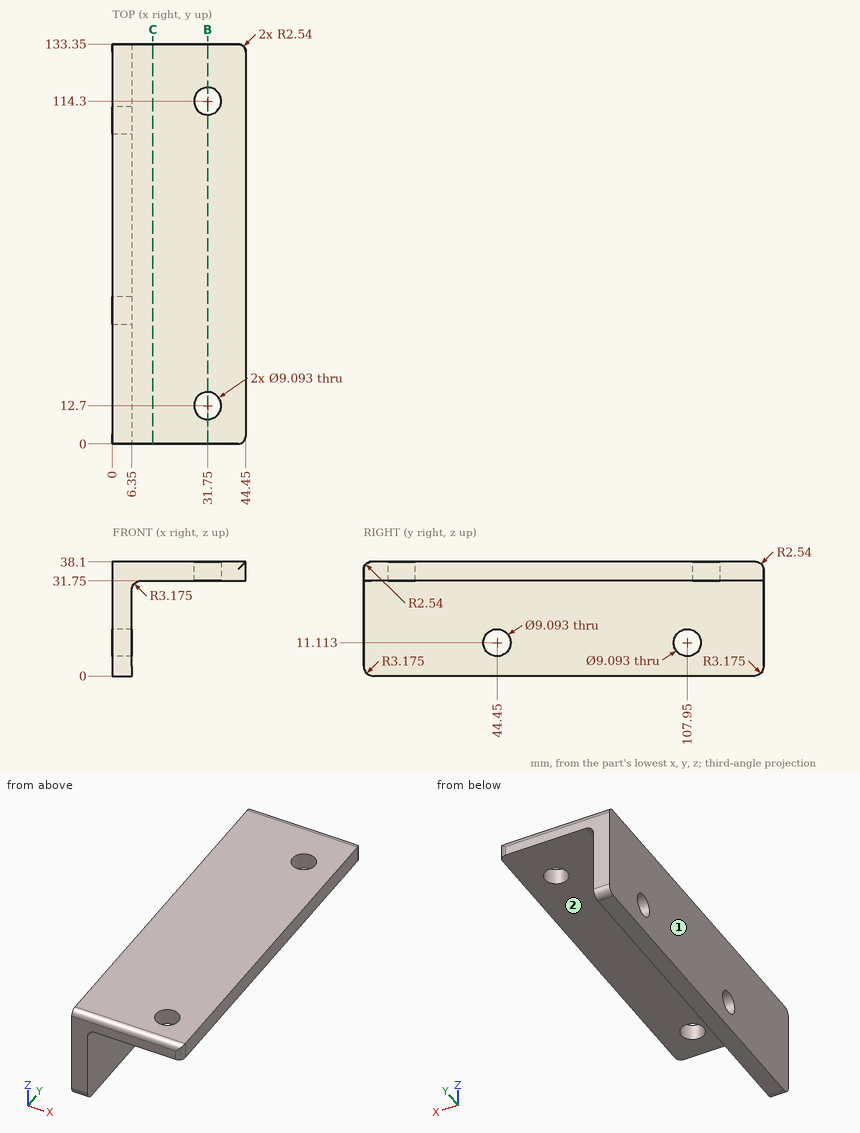
Verification items for this drawing (mm, ordinates from the low corner). A direction names the side the tool comes from. Coordinates: 2 decimals unless noted, no trailing zeros. Order: outer loops, then holes, each group sorted by start corner. A loop starts at its lowest first (then second) coordinate and runs counter-clockwise, first axis right, second up. Notation, with made-up numbers: (45, 74.25) -> (103, 74.25) arc R20 ccw to (103, 90.25) -> close; hole circle Ø7 at (-37.5, 46.5). An arc over 180 degrees is marked (long way). Answer as CSV lines item,"result". Start each with the question number.
1) Cross-section at B-B, the plane x = 31.75. Record the boundary of the cut face in (y, z).
2) Set-up check for the marked faces 1 and 2: record each of +Z, -Z, +X, -X, +Y, -Y from which the full face is reachable in a straight line by a thin tool's end or side.
3) Cross-section at C-C, the plane x = 13.5. Record the boundary of the cut face in (y, z), then the cut area to 3 significant figures.
4) Material ranges on L1, parallel to Z at x = 4.25, y = 107.95 (1 decimal); L2, parallel to Y at x = 31.75, z = 36.75 (1 decimal); L3, parallel to Y at x = 31, z = 36 (1 decimal), recorded low to high. Write a range as [from, to].
5) Gauge pin test, flat ends, axial feed: pin 1 Ø1.5 at (x, y) = (13, 109) entering from -Z; pin 2 Ø10 at (x, z) = (23, 26.5) entering from +Y; pin 3 Ø8.5 at (y, z) = (64.5, 7) entering from +X. Record the tip position at first contact, or that the pin passes through.
Conclusion:
1,outline,"(0, 31.75) -> (8.15, 31.75) -> (8.15, 38.1) -> (2.54, 38.1) arc R2.54 ccw to (0, 35.56) -> close; (17.25, 31.75) -> (109.75, 31.75) -> (109.75, 38.1) -> (17.25, 38.1) -> close; (118.85, 31.75) -> (133.35, 31.75) -> (133.35, 35.56) arc R2.54 ccw to (130.81, 38.1) -> (118.85, 38.1) -> close"
2,face 1,"+Z, -Z, -X, +Y, -Y"
2,face 2,"-Z, +X, +Y, -Y"
3,outline,"(0, 31.75) -> (133.35, 31.75) -> (133.35, 35.56) arc R2.54 ccw to (130.81, 38.1) -> (2.54, 38.1) arc R2.54 ccw to (0, 35.56) -> close"
3,area,"844 mm²"
4,L1,"z = [0, 6.6], [15.7, 38.1]"
4,L2,"y = [0.3, 8.2], [17.2, 109.8], [118.8, 133.1]"
4,L3,"y = [0, 8.2], [17.2, 109.8], [118.8, 133.3]"
5,pin 1,"stops at z = 31.75"
5,pin 2,"passes through"
5,pin 3,"stops at x = 6.35"
